```python
from build123d import *

# Parameters (mm, degrees)
SKETCH1_R                = 30
BOSS_EXTRUDE1_DEPTH      = 60
CHAMFER1_SIZE            = 5
CUT_EXTRUDE1_DEPTH       = 25
CIRPATTERN1_COUNT        = 6
SKETCH3_R                = 20
CUT_EXTRUDE2_DEPTH       = 30
SKETCH5_R                = 12.5
CUT_EXTRUDE3_DEPTH       = 91
CHAMFER2_SIZE            = 5
MIRROR1_COPY_1_DEPTH     = 25
MIRROR1_COPY_2_DEPTH     = 25
MIRROR1_COPY_3_DEPTH     = 25
MIRROR1_COPY_4_DEPTH     = 25
MIRROR1_COPY_5_DEPTH     = 25
CHAMFER2_OF_MIRROR1_SIZE = 5
BOSS_EXTRUDE2_REACH      = 82
BOSS_EXTRUDE2_END_RADIUS = 30
CUT_EXTRUDE4_REACH       = 82
CUT_EXTRUDE4_END_RADIUS  = 17
SKETCH8_R                = 7.5


with BuildPart() as part:
    # Sketch1 → Boss-Extrude1 (new body, symmetric)
    with BuildSketch(Plane(origin=(0, 0, 0), x_dir=(0, 0, -1), z_dir=(1, 0, 0))):
        Circle(SKETCH1_R)
    extrude(amount=BOSS_EXTRUDE1_DEPTH, both=True)

    # Chamfer1
    chamfer1_edges = [part.edges().sort_by_distance(p)[0] for p in [
        (-60, 0, 30),
        (60, 0, 30),
    ]]
    chamfer(chamfer1_edges, length=CHAMFER1_SIZE)

    # Sketch2 → Cut-Extrude1 (cut)
    with BuildSketch(Plane(origin=(60, 0, 0), x_dir=(0, 0, -1), z_dir=(1, 0, 0))):
        with BuildLine():
            Line((28, 10.770329614), (28, -10.770329614))
            ThreePointArc((28, -10.770329614), (30, 0), (28, 10.770329614))
        make_face()
    cut_extrude1 = extrude(amount=-CUT_EXTRUDE1_DEPTH, mode=Mode.SUBTRACT)

    # CirPattern1: Cut-Extrude1 ×6 about axis
    cirpattern1_axis = Axis((0, 0, 0), (1, 0, 0))
    for i in range(1, CIRPATTERN1_COUNT):
        add(cut_extrude1.rotate(cirpattern1_axis, i * 360 / CIRPATTERN1_COUNT), mode=Mode.SUBTRACT)

    # Sketch3 → Cut-Extrude2 (cut)
    with BuildSketch(Plane(origin=(60, 0, 0), x_dir=(0, 0, -1), z_dir=(1, 0, 0))):
        Circle(SKETCH3_R)
    cut_extrude2 = extrude(amount=-CUT_EXTRUDE2_DEPTH, mode=Mode.SUBTRACT)

    # Sketch5 → Cut-Extrude3 (cut, through all)
    with BuildSketch(Plane(origin=(30, 0, 0), x_dir=(0, 0, -1), z_dir=(1, 0, 0))):
        Circle(SKETCH5_R)
    extrude(amount=-CUT_EXTRUDE3_DEPTH, mode=Mode.SUBTRACT)

    # Sketch4 → Cut-Revolve1 (revolve, cut)
    with BuildSketch(Plane.XY):
        with BuildLine():
            Line((0, 17), (0, -17))
            ThreePointArc((0, -17), (17, 0), (0, 17))
        make_face()
    revolve(axis=Axis((0, 40.549893096, 0), (0, -1, 0)), mode=Mode.SUBTRACT)

    # Chamfer2
    chamfer2_edges = [part.edges().sort_by_distance(p)[0] for p in [
        (30, 0, 12.5),
    ]]
    chamfer(chamfer2_edges, length=CHAMFER2_SIZE)

    # Mirror1: Cut-Extrude1, Cut-Extrude2 across plane
    add(cut_extrude1.mirror(Plane(origin=(0, 0, 0), x_dir=(0, 0, 1), z_dir=(1, 0, 0))), mode=Mode.SUBTRACT)
    add(cut_extrude2.mirror(Plane(origin=(0, 0, 0), x_dir=(0, 0, 1), z_dir=(1, 0, 0))), mode=Mode.SUBTRACT)

    # Mirror1 copy 1 sketch → Mirror1 copy 1 (cut)
    with BuildSketch(Plane(origin=(-60, 0, 0), x_dir=(0, 0.866025404, -0.5), z_dir=(-1, 0, 0))):
        with BuildLine():
            Line((28, -10.770329614), (28, 10.770329614))
            ThreePointArc((28, 10.770329614), (30, 0), (28, -10.770329614))
        make_face()
    extrude(amount=-MIRROR1_COPY_1_DEPTH, mode=Mode.SUBTRACT)

    # Mirror1 copy 2 sketch → Mirror1 copy 2 (cut)
    with BuildSketch(Plane(origin=(-60, 0, 0), x_dir=(0, 0.866025404, 0.5), z_dir=(-1, 0, 0))):
        with BuildLine():
            Line((28, -10.770329614), (28, 10.770329614))
            ThreePointArc((28, 10.770329614), (30, 0), (28, -10.770329614))
        make_face()
    extrude(amount=-MIRROR1_COPY_2_DEPTH, mode=Mode.SUBTRACT)

    # Mirror1 copy 3 sketch → Mirror1 copy 3 (cut)
    with BuildSketch(Plane.ZY.offset(60)):
        with BuildLine():
            Line((28, -10.770329614), (28, 10.770329614))
            ThreePointArc((28, 10.770329614), (30, 0), (28, -10.770329614))
        make_face()
    extrude(amount=-MIRROR1_COPY_3_DEPTH, mode=Mode.SUBTRACT)

    # Mirror1 copy 4 sketch → Mirror1 copy 4 (cut)
    with BuildSketch(Plane(origin=(-60, 0, 0), x_dir=(0, -0.866025404, 0.5), z_dir=(-1, 0, 0))):
        with BuildLine():
            Line((28, -10.770329614), (28, 10.770329614))
            ThreePointArc((28, 10.770329614), (30, 0), (28, -10.770329614))
        make_face()
    extrude(amount=-MIRROR1_COPY_4_DEPTH, mode=Mode.SUBTRACT)

    # Mirror1 copy 5 sketch → Mirror1 copy 5 (cut)
    with BuildSketch(Plane(origin=(-60, 0, 0), x_dir=(0, -0.866025404, -0.5), z_dir=(-1, 0, 0))):
        with BuildLine():
            Line((28, -10.770329614), (28, 10.770329614))
            ThreePointArc((28, 10.770329614), (30, 0), (28, -10.770329614))
        make_face()
    extrude(amount=-MIRROR1_COPY_5_DEPTH, mode=Mode.SUBTRACT)

    # Chamfer2 of Mirror1
    chamfer2_of_mirror1_edges = [part.edges().sort_by_distance(p)[0] for p in [
        (-30, 0, 12.5),
    ]]
    chamfer(chamfer2_of_mirror1_edges, length=CHAMFER2_OF_MIRROR1_SIZE)

    # Boss-Extrude2: up to this cylinder (the profile starts outside it)
    boss_extrude2_end = Plane(origin=(0.286485, 0, 0), z_dir=(-1, 0, 0)) * Cylinder(BOSS_EXTRUDE2_END_RADIUS, 225, mode=Mode.PRIVATE)
    # Sketch6 → Boss-Extrude2 (add, up to the surface)
    with BuildSketch(Plane(origin=(0, 50, 0), x_dir=(1, 0, 0), z_dir=(0, 1, 0)), mode=Mode.PRIVATE) as boss_extrude2_sk1:
        with BuildLine():
            Line((17.860571099, 9), (25.025354797, 9))
            Line((25.025354797, 9), (25.025354797, 14))
            Line((25.025354797, 14), (5.176380902, 19.318516526))
            ThreePointArc((5.176380902, 19.318516526), (-14.142135624, 14.142135624), (-19.318516526, -5.176380902))
            Line((-19.318516526, -5.176380902), (-14, -25.025354797))
            Line((-14, -25.025354797), (-9, -25.025354797))
            Line((-9, -25.025354797), (-9, -17.860571099))
            ThreePointArc((-9, -17.860571099), (14.142135624, -14.142135624), (17.860571099, 9))
        make_face()
    boss_extrude2_tool1 = extrude(boss_extrude2_sk1.sketch, amount=-BOSS_EXTRUDE2_REACH, mode=Mode.PRIVATE) - boss_extrude2_end
    add(boss_extrude2_tool1.solids().sort_by_distance((0.286485, 50, 0.286485))[0])

    # Cut-Extrude4: up to this sphere (the profile starts outside it)
    cut_extrude4_end = Location((0, 0, 0)) * Sphere(CUT_EXTRUDE4_END_RADIUS, mode=Mode.PRIVATE)
    # Sketch8 → Cut-Extrude4 (cut, up to the surface)
    with BuildSketch(Plane(origin=(0, 50, 0), x_dir=(1, 0, 0), z_dir=(0, 1, 0)), mode=Mode.PRIVATE) as cut_extrude4_sk1:
        with Locations(Location((0, 0, 0), (0, 0, 270))):  # turned: the seam where the file's is
            Circle(SKETCH8_R)
    cut_extrude4_tool1 = extrude(cut_extrude4_sk1.sketch, amount=-CUT_EXTRUDE4_REACH, mode=Mode.PRIVATE) - cut_extrude4_end
    add(cut_extrude4_tool1.solids().sort_by_distance((0, 50, 0))[0], mode=Mode.SUBTRACT)


solid = part.part
```
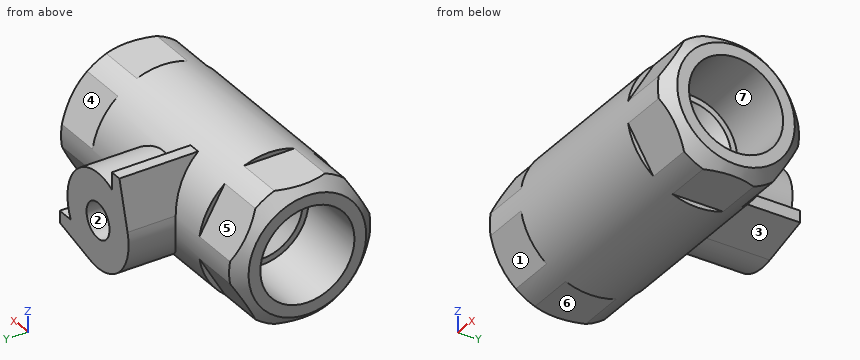
Can you work these out from the model? Positions are in its coordinate system, mm. Face numbers are marked on the shaded views. A direction names the side the tool comes from. Give positions to 0.01 mm unless a question says otherwise; leave off trailing zeros. Loops run counter-clockwise (first coordinate to the right, second up) from the corner with the lowest first, then second, coordinate; pieces in that order, holes last. Notation, with made-up numbers: M 52,30 L 105,30 A23 ccw 105,61 Z; hole C 32.25,-15 d10. An arc over 180 degrees is marked long. Use one line per item in the form item = value. Start each with the question number.
(1) Please list where these lines run through material, in increasing order: line 1 (Z direction, x = 0, y = 41); line 2 (Y direction, x = -36.25, z = 0); line 3 (Y direction, x = -17.5, z = 0).
(2) On a 3-axis mill with a long thin cutter (end or side, diameter ignored), from which of +Z, -Z, +X, -X, +Y, -Y can I reach the whole of each face in a straight line? I mean the marked faces 1, 2, 3 and 4. Say none if no direction works.
(3) I want a section at C-C, the plane x = 38. Write out the boundary of the cut face in (y, z), and give its area (3 significant figures).
(4) Thinking about a two-plate mould opening in Z: for the marked faces 5, 6 and 7, which applies, released by +Z, released by -Z, zero draft, split by the parting line, or undercut?
(5) I want a section at B-B, the plane x = 0. Write out the boundary of the cut face in (y, z).
(6) I'm going to push flat-ended pins straight in: P1, Ø1, axis at x = 42.5, z = -13, coming from the -Y side; P2, Ø12, axis at y = 8, z = 1, coming from the +X side; P3, Ø1, axis at x = -26.5, y = -8.5, coming from the -Z side; P4, Ø22.5, axis at y = 0, z = 0, coming from the -X side. Where does each tip first touch, or does it pass through?
(7) I want a section at A-A, the plane y = 39. Write out the boundary of the cut face in (x, z).
(8) I want a section at D-D, the plane z = -6. State how many separate pieces and enclosed holes the cut face has, and give its area (3 significant figures).
Worked out:
q1.line_1 = -20 to -7.5, 7.5 to 20
q1.line_2 = -30 to -20, 20 to 30
q1.line_3 = -30 to -12.5, 12.5 to 50
q2.face_1 = -Z, -X, -Y
q2.face_2 = +Y
q2.face_3 = -Z, +X, +Y
q2.face_4 = +Z, +X, +Y
q3.outline = M -29.63,-4.67 L -18.86,-23.33 A30 ccw -10.77,-28 L 10.77,-28 A30 ccw 18.86,-23.33 L 29.63,-4.67 A30 ccw 29.63,4.67 L 18.86,23.33 A30 ccw 10.77,28 L -10.77,28 A30 ccw -18.86,23.33 L -29.63,4.67 A30 ccw Z; hole C 0,0 d40
q3.area = 1,400 mm²
q4.face_5 = released by +Z
q4.face_6 = released by -Z
q4.face_7 = undercut
q5.outline = M 15.26,-7.5 A17 cw long 15.26,7.5 L 50,7.5 L 50,20 L 22.36,20 A30 ccw long 22.36,-20 L 50,-20 L 50,-7.5 Z
q6.P1 = -25.11
q6.P2 = 26.56
q6.P3 = -28.91
q6.P4 = through
q7.outline = M -19.32,5.18 A20 ccw 5.18,-19.32 L 25.03,-14 L 25.03,-9 L 17.86,-9 A20 ccw -9,17.86 L -9,25.03 L -14,25.03 Z; hole C 0,0 d15
q8.separate_pieces = 3
q8.enclosed_holes = 0
q8.area = 3,620 mm²
